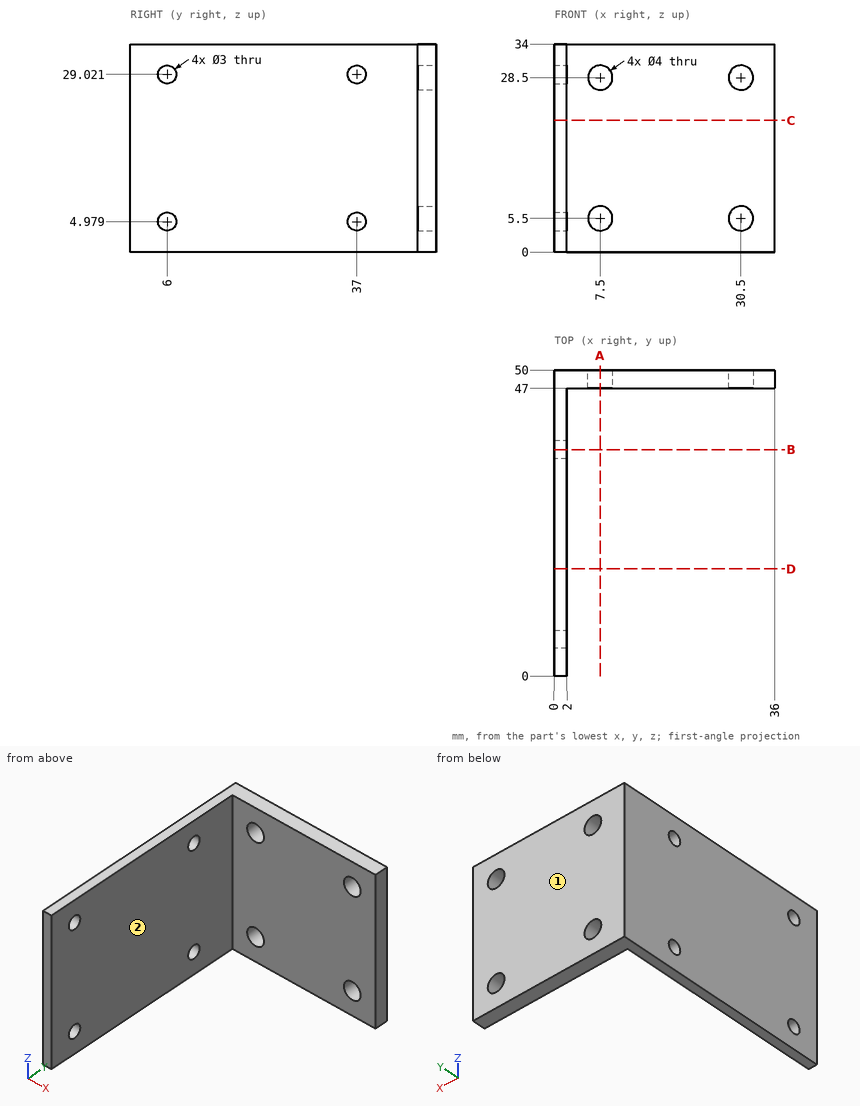
Can you work these out from the drawing? Everything is in mm from the part's minimum corner. A direction names the side the tool comes from. Coordinates: 2 decimals unless noted, no trailing zeros. Loops run counter-clockwise (first coordinate to the right, second up) from the corner with the lowest first, then second, coordinate; pieces in that order, holes last. Notation, with made-up numbers: (58, 78.25) - (114, 78.25) arc R4 cw to (114, 83.25) - close; hole circle Ø11 at (-32, 62). An arc over 180 degrees is marked (long way). Use a Markdown table: item, result.
Item 1: Will these pins go through, and if not, where does the flat tip stop? pin 1 (12 mm diameter, centred on y = 42, z = 15, fed in from -X); pin 2 (4 mm diameter, centred on y = 34, z = 26.5, fed in from +X); pin 3 (2.5 mm diameter, centred on y = 37, z = 29.02, fed in from +X); pin 4 (17 mm diameter, centred on x = 12.5, z = 11, fed in from -Y).
Numbers:
| item | result |
|---|---|
| pin 1 | stops at x = 0 |
| pin 2 | stops at x = 2 |
| pin 3 | passes through |
| pin 4 | stops at y = 47 |
Item 2: I want a section at B-B on y = 37. Please give me the cut outline in (x, z).
Numbers:
| item | result |
|---|---|
| outline | (0, 0) - (2, 0) - (2, 3.48) - (0, 3.48) - close; (0, 6.48) - (2, 6.48) - (2, 27.52) - (0, 27.52) - close; (0, 30.52) - (2, 30.52) - (2, 34) - (0, 34) - close |
Item 3: I want a section at A-A on x = 7.5. Please give me the cut outline in (y, z).
Numbers:
| item | result |
|---|---|
| outline | (47, 0) - (50, 0) - (50, 3.5) - (47, 3.5) - close; (47, 7.5) - (50, 7.5) - (50, 26.5) - (47, 26.5) - close; (47, 30.5) - (50, 30.5) - (50, 34) - (47, 34) - close |
Item 4: For the marked faces 1 and 2, which set-ups out of +Z, -Z, +X, -X, +Y, -Y let a thin tool reach every point of the face, with its end or its side?
Numbers:
| item | result |
|---|---|
| face 1 | +Z, -Z, +X, -X, +Y |
| face 2 | +Z, -Z, +X, -Y |
Item 5: If I drill on probe 1 along Z at (x, y) = (0.8, 6); probe 2 along Z at (x, y) = (30.5, 47.95); probe 3 along Y at (x, z) = (21, 28.5), over which ranges is the centre line in solid material (lowest first)? Write a range as from..to.
Numbers:
| item | result |
|---|---|
| probe 1 | z = 0..3.48, 6.48..27.52, 30.52..34 |
| probe 2 | z = 0..3.5, 7.5..26.5, 30.5..34 |
| probe 3 | y = 47..50 |
Item 6: I want a section at C-C on z = 21.5. Please give me the cut outline in (x, y), and give its area (3 significant figures).
Numbers:
| item | result |
|---|---|
| outline | (0, 0) - (2, 0) - (2, 47) - (36, 47) - (36, 50) - (0, 50) - close |
| area | 202 mm2 |
Item 7: I want a section at D-D on y = 17.5. Please give me the cut outline in (x, z).
Numbers:
| item | result |
|---|---|
| outline | (0, 0) - (2, 0) - (2, 34) - (0, 34) - close |
